Autodesk Inventor part; units mm, degrees
ref_plane "YZ Plane" through (0, 0, 0) normal (1, 0, 0) x (0, 1, 0)
ref_plane "XZ Plane" through (0, 0, 0) normal (0, 1, 0) x (-1, 0, 0)
ref_plane "XY Plane" through (0, 0, 0) normal (0, 0, 1) x (1, 0, 0)
ref_plane "Work Plane1" through (0, 0, -17.5) normal (0, 0, 1) x (1, 0, 0)
sketch "Sketch1" plane through (0, 0, -17.5) normal (0, 0, 1) x (1, 0, 0)
  line L0 (-31, 0) -> (-31, 120) construction
  line L1 (3, 17.5) -> (-715, 17.5) construction
  line L2 (-39, 17.5) -> (-81, 17.5)
  line L3 (-81, 17.5) -> (-81, 27.5)
  line L4 (-41, 47.5) -> (-31, 47.5)
  line L5 (-31, 47.5) -> (-31, 25.5)
  line L6 (-31, 25.5) -> (-39, 17.5)
  line L7 (-81, 27.5) -> (-41, 47.5)
  point P0 (0, 0)
  point P1 (-31, 17.5)
  point P2 (-81, 47.5)
  dimension "d0" = 50
  dimension "d1" = 30
  dimension "d2" = 8
  dimension "d3" = 8
  dimension "d4" = 20
  dimension "d5" = 40
extrude "Extrusion1" add sketch "Sketch1" along normal mid plane 10
properties part number "Gusset" material "Steel, Alloy"
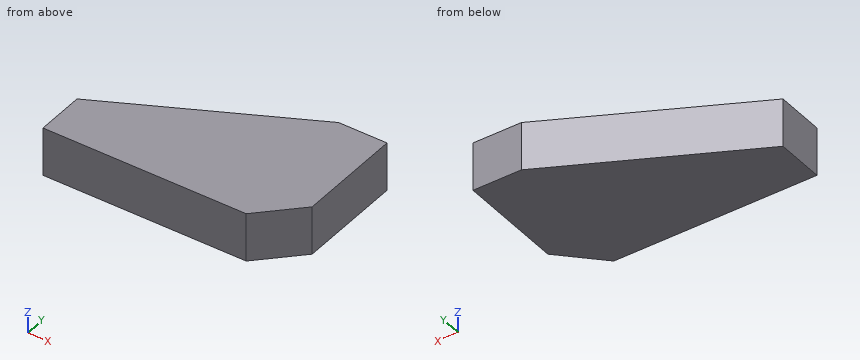
Here's how the part is built. I have some questions about the finished solid (model axes, mm). Round coordinates to 2 decimals unless told otherwise and drop trailing zeros. Loops run counter-clockwise (first coordinate to the right, second up) from the corner with the lowest first, then second, coordinate; pieces in that order, holes last. Notation, with made-up numbers: M 48.25,71 L 77.25,71 A31 ccw 77.25,103 Z; hole C -17,-38.75 d7. An arc over 180 degrees is marked long. Write each question's results on one line, items separated by ' | '. Start each with the question number.
(1) Will these pins go through, and if not, where does the flat tip stop? P1, Ø10, axis at x = -61, y = 44, coming from the -Z side; P2, Ø4, axis at y = 30, z = -16, coming from the -X side.
(2) I want a section at C-C (x = -49). Please give me the cut outline in (y, z), then the cut area to 3 significant figures.
(3) I want a section at B-B (y = 22). Please give me the cut outline in (x, z).
(4) I want a section at A-A (z = -16.75). Please give me the cut outline in (x, y).
(5) If I drill on probe 1 along X at (y, z) = (28, -19.5); probe 2 along Y at (x, z) = (-61, -18); probe 3 along X at (y, z) = (21, -21.25), over which ranges is the centre line in solid material (lowest first)? Write a range as from..to.
Solved:
1) P1: passes through | P2: stops at x = -80
2) outline: M 17.5,-22.5 L 43.5,-22.5 L 43.5,-12.5 L 17.5,-12.5 Z | area: 260 mm²
3) outline: M -81,-22.5 L -34.5,-22.5 L -34.5,-12.5 L -81,-12.5 Z
4) outline: M -81,17.5 L -39,17.5 L -31,25.5 L -31,47.5 L -41,47.5 L -81,27.5 Z
5) probe 1: x = -80..-31 | probe 2: y = 17.5..37.5 | probe 3: x = -81..-35.5
